```python
from build123d import *

# Parameters (mm, degrees)
SKETCH1_W              = 100
SKETCH1_H              = 50
BASE_FLANGE1_DEPTH     = 2.5
SKETCHED_START         = -25
SKETCHED_BEND3_DEPTH   = 50
SKETCHED_BEND3_2_DEPTH = 50


# Read off the part's stored shape, not the designer's step: Sketched Bend3
# Sheet-metal steps are written as plain solids
with BuildPart() as part:
    # Sketch1 → Base-Flange1 (new body)
    with BuildSketch(Plane(origin=(0, 0, 0), x_dir=(1, 0, 0), z_dir=(0, 1, 0))):
        Rectangle(SKETCH1_W, SKETCH1_H)
    extrude(amount=-BASE_FLANGE1_DEPTH)

    # Sketched Bend3 outline → Sketched Bend3 (cut)
    with BuildSketch(Plane.XY.offset(SKETCHED_START)):
        with BuildLine():
            Line((50, 0), (6.071738955, 0))
            Line((6.071738955, 0), (0.92655011, -2.214803911))
            ThreePointArc((0.92655011, -2.214803911), (0.249167174, -2.427959574), (-0.457298081, -2.5))
            Line((-0.457298081, -2.5), (50, -2.5))
            Line((50, -2.5), (50, 0))
        make_face()
    extrude(amount=SKETCHED_BEND3_DEPTH, mode=Mode.SUBTRACT)

    # Sketched Bend3 2 outline → Sketched Bend3 2 (add)
    with BuildSketch(Plane.XY.offset(SKETCHED_START)):
        with BuildLine():
            Line((46.432284933, 17.373647068), (45.443821939, 19.669935575))
            Line((45.443821939, 19.669935575), (-0.061912883, 0.081484597))
            ThreePointArc((-0.061912883, 0.081484597), (-0.255450865, 0.020582979), (-0.457298081, 0))
            Line((-0.457298081, 0), (6.071738955, 0))
            Line((6.071738955, 0), (46.432284933, 17.373647068))
        make_face()
    extrude(amount=SKETCHED_BEND3_2_DEPTH)


solid = part.part
```
Read the model definition and answer for the solid it produces. Units are mm, in the model's axes. A direction names the side the tool comes from. Give positions to 0.01 mm unless a question says otherwise; leave off trailing zeros. Order: outer loops, then holes, each group sorted by start corner. A loop starts at its lowest first (then second) coordinate and runs counter-clockwise, first axis right, second up. Notation, with made-up numbers: (-1, 81.25) -> (56, 81.25) arc R32 ccw to (56, 108.25) -> close; hole circle Ø5 at (65, 18). An arc over 180 degrees is marked (long way). One line per item, written item: value. Start each with the question number.
(1) Straight lines are drawn through the part: L1, parallel to Y at x = -26, z = -16; L2, parallel to Y at x = 37, z = 20; L3, parallel to X at y = 17.5, z = 10. For each, find the intervals that lie inside material, in ascending order.
(2) Flat-ended cylindrical pins translate along their axes: P1, Ø25, axis at x = -25, z = 1.5, coming from the +Y side; P2, Ø6, axis at y = 14.5, z = -1.5, coming from the -X side; P3, Ø12, axis at x = 14, z = 17.5, coming from the -Y side. Find the tip coordinate at first contact, or state that the pin passes through.
(3) The part is cut by section C-C (y = 13.5). Determine the outline of the cut face in (x, z).
(4) The part is cut by section A-A (z = -9). Determine the outline of the cut face in (x, y), and give its area (3 significant figures).
(5) A tool of negligible diameter and unlimited length cuts with its end or side. For faces 1 (the flat face through (-26, -2.5, 0)), 2 (the flat face through (-26, 0, 0)), from which of +Z, -Z, +X, -X, +Y, -Y can it reach the whole face along a straight path? Write none if from no direction.
(6) The part is cut by section B-B (x = -14). Determine the outline of the cut face in (y, z).
Taken from the geometry:
1. L1: -2.5 to 0
1. L2: 13.31 to 16.04
1. L3: 40.4 to 46.38
2. P1: y = 0
2. P2: x = 26.46
2. P3: y = 0.83
3. outline: (31.11, -25) -> (37.43, -25) -> (37.43, 25) -> (31.11, 25) -> close
4. outline: (-50, -2.5) -> (-0.46, -2.5) arc R3.5 ccw to (0.93, -2.21) -> (46.43, 17.37) -> (45.44, 19.67) -> (-0.06, 0.08) arc R1 cw to (-0.46, 0) -> (-50, 0) -> close
4. area: 250 mm^2
5. face 1: +Z, -Z, +X, -X, -Y
5. face 2: +Z, -Z, -X, +Y
6. outline: (-2.5, -25) -> (0, -25) -> (0, 25) -> (-2.5, 25) -> close
